Design review of the part built by this model. Coordinates are the model's own, in mm. Coordinates: 2 decimals unless noted, no trailing zeros. Write each loop counter-clockwise with the first axis right and the second up, starting at its lowest first coordinate (ties: lowest second). Pieces come first, ordered by that corner, then holes. Notation, with made-up numbers: (23, 36.25) - (28, 36.25) arc R14 ccw to (28, 40.25) - close; hole circle Ø1 at (49.25, 12.5). An arc over 180 degrees is marked (long way). Answer as CSV lines item,"result". Start each with the question number.
Q1. We need section B-B (x = 5.75). Write out the cut boundary in (y, z).
Q2. Clearance check with a flat-ended pin moving along its axis: pin 1 (3.5 mm diameter, centred on x = 0, y = -17.63, fed in from -Z). State where the tip first meets the part, or that it passes through.
Q3. For line 1 along Y through (x, z) = (1.5, 0.75); line 2 along Y through (x, z) = (1, 0.9); line 3 along Y through (x, z) = (-4.5, 0.85), list the stretches that pass through material, from the lowest coordinate up. Write a range as [from, to].
Q4. We need section C-C (x = -5.5). Write out the cut boundary in (y, z).
Q5. We need section A-A (z = 0.9). State how many separate pieces and enclosed holes the cut face has, plus the area to 3 significant figures.
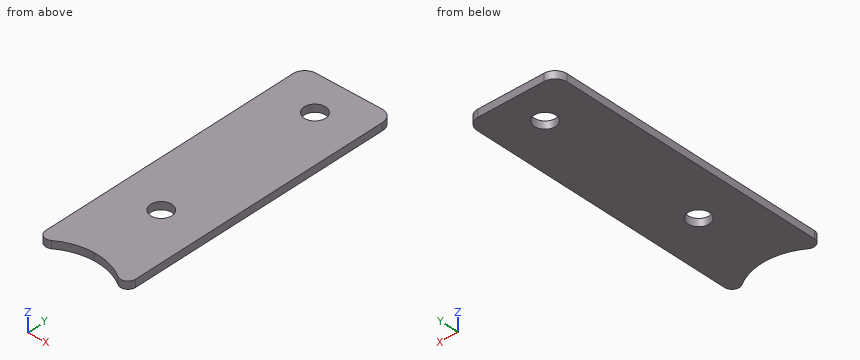
from build123d import *

# Parameters (mm, degrees)
SKETCH1_W            = 19.05
SKETCH1_H            = 50.8
BOSS_EXTRUDE1_DEPTH  = 1.5875
M4_CLEARANCE_HOLE1_D = 4.5
SKETCH4_W            = 19.05
SKETCH4_H            = 7.62
BOSS_EXTRUDE2_DEPTH  = 1.5875
FILLET1_R            = 2.54
BOSS_EXTRUDE3_DEPTH  = 1.5875
FILLET2_R            = 1.5875


with BuildPart() as part:
    # Sketch1 → Boss-Extrude1 (new body)
    with BuildSketch(Plane.XY):
        Rectangle(SKETCH1_W, SKETCH1_H)
    extrude(amount=BOSS_EXTRUDE1_DEPTH)

    # M4 Clearance Hole1 (through all)
    with Locations(Plane.XY.offset(1.5875)):
        with Locations((0, 17.6276), (0, -17.6276)):
            Hole(M4_CLEARANCE_HOLE1_D / 2)

    # Sketch4 → Boss-Extrude2 (add)
    with BuildSketch(Plane.XY.offset(1.5875)):
        with Locations((0, -29.21)):
            Rectangle(SKETCH4_W, SKETCH4_H)
    extrude(amount=-BOSS_EXTRUDE2_DEPTH)

    # Fillet1
    fillet1_edges = [part.edges().sort_by_distance(p)[0] for p in [
        (-9.525, 25.4, 0.79375),
        (9.525, 25.4, 0.79375),
    ]]
    fillet(fillet1_edges, radius=FILLET1_R)

    # Sketch5 → Boss-Extrude3 (add)
    with BuildSketch(Plane.XY.offset(1.5875)):
        with BuildLine():
            Line((1.5e-08, -33.02), (-9.525, -33.02))
            Line((-9.525, -33.02), (-9.525, -37.319739587))
            ThreePointArc((-9.525, -37.319739587), (-5.225260406, -34.144739584), (1.5e-08, -33.02))
        make_face()
        with BuildLine():
            Line((9.525, -33.02), (1.5e-08, -33.02))
            ThreePointArc((1.5e-08, -33.02), (5.225260419, -34.14473959), (9.525, -37.319739587))
            Line((9.525, -37.319739587), (9.525, -33.02))
        make_face()
    extrude(amount=-BOSS_EXTRUDE3_DEPTH)

    # Fillet2
    fillet2_edges = [part.edges().sort_by_distance(p)[0] for p in [
        (-9.525, -37.319739587, 0.79375),
        (9.525, -37.319739587, 0.79375),
    ]]
    fillet(fillet2_edges, radius=FILLET2_R)


solid = part.part
Results list:
1,outline,"(-34.4, 0) - (25.4, 0) - (25.4, 1.59) - (-34.4, 1.59) - close"
2,pin 1,"passes through"
3,line 1,"y = [-33.11, -19.3], [-15.95, 15.95], [19.3, 25.4]"
3,line 2,"y = [-33.06, -19.64], [-15.61, 15.61], [19.64, 25.4]"
3,line 3,"y = [-33.84, 25.4]"
4,outline,"(-34.27, 0) - (25.4, 0) - (25.4, 1.59) - (-34.27, 1.59) - close"
5,separate pieces,"1"
5,enclosed holes,"2"
5,area,"1,100 mm2"
